Design review of the part built by this model. Coordinates are the model's own, in mm. Face numbers are marked on the shaded views. A direction names the side the tool comes from. Coordinates: 2 decimals unless noted, no trailing zeros. Loops run counter-clockwise (first coordinate to the right, second up) from the corner with the lowest first, then second, coordinate; pieces in that order, holes last. Notation, with made-up numbers: (-26.75, -22.5) -> (-9.75, -22.5) arc R31 ccw to (-9.75, 4.5) -> close; hole circle Ø2 at (35.25, 72.25). An arc over 180 degrees is marked (long way). Answer in a Markdown table with one row per item.
```python
from build123d import *

# Parameters (mm, degrees)
EXTRUDE_1_DEPTH = 20
EXTRUDE_2_DEPTH = 2.5
SKETCH_3_W      = 12
SKETCH_3_H      = 4
EXTRUDE_3_DEPTH = 10
FILLET_1_R      = 2


with BuildPart() as part:
    # 草图1 → 凸台-拉伸1 (new body)
    with BuildSketch(Plane(origin=(0, 0, 0), x_dir=(1, 0, 0), z_dir=(0, 1, 0))):
        Polygon((35, 66), (66, 35), (66, 0), (0, 0), (0, 66), align=None)
    extrude(amount=EXTRUDE_1_DEPTH)

    # 草图2 → 凸台-拉伸2 (add)
    with BuildSketch(Plane(origin=(50.5, 0, -50.5), x_dir=(-0.7071067811865475, 0, -0.7071067811865477), z_dir=(0.7071067811865477, 0, -0.7071067811865475))):
        with BuildLine():
            Line((15.5, 15), (15.5, 5))
            ThreePointArc((15.5, 5), (14.621320344, 2.878679656), (12.5, 2))
            Line((12.5, 2), (-12.5, 2))
            ThreePointArc((-12.5, 2), (-14.621320344, 2.878679656), (-15.5, 5))
            Line((-15.5, 5), (-15.5, 15))
            ThreePointArc((-15.5, 15), (-14.621320344, 17.121320344), (-12.5, 18))
            Line((-12.5, 18), (12.5, 18))
            ThreePointArc((12.5, 18), (14.621320344, 17.121320344), (15.5, 15))
        make_face()
    extrude(amount=EXTRUDE_2_DEPTH)

    # 草图3 → 凸台-拉伸3 (add)
    with BuildSketch(Plane(origin=(52.267766953, 0, -52.267766953), x_dir=(-0.7071067811865476, 0, -0.7071067811865476), z_dir=(0.7071067811865476, 0, -0.7071067811865476))):
        with Locations((0, 10)):
            Rectangle(SKETCH_3_W, SKETCH_3_H)
    extrude(amount=EXTRUDE_3_DEPTH)

    # 圆角1
    fillet_1_edges = [part.edges().sort_by_distance(p)[0] for p in [
        (66, 20, -17.5),
        (50.5, 20, -50.5),
        (17.5, 20, -66),
        (0, 20, -33),
        (17.5, 0, -66),
        (50.5, 0, -50.5),
        (66, 0, -17.5),
        (33, 0, 0),
        (0, 0, -33),
        (33, 20, 0),
        (0, 10, -66),
        (66, 10, 0),
        (0, 10, 0),
    ]]
    fillet(fillet_1_edges, radius=FILLET_1_R - 0.0001)  # a hair under: the kernel refuses the full size


solid = part.part
```
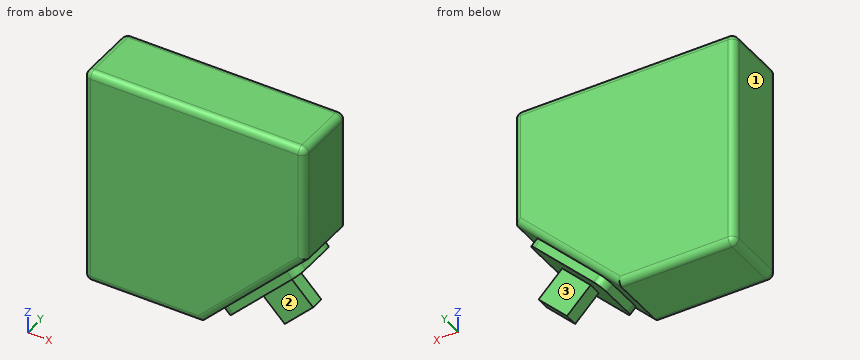
(1) Take a section at B-B on y = 13.5. Give the boundary of the cut face in (x, z), and give its area (3 significant figures).
Evaluation:
| item | result |
|---|---|
| outline | (0, -64) arc R2 ccw to (2, -66) -> (35, -66) -> (39.54, -61.46) -> (41.31, -63.23) -> (63.23, -41.31) -> (61.46, -39.54) -> (66, -35) -> (66, -2) arc R2 ccw to (64, 0) -> (2, 0) arc R2 ccw to (0, -2) -> close |
| area | 3,950 mm² |
(2) Tool access review of the marked faces 1, 2 and 3: name each direction out of +Z, -Z, +X, -X, +Y, -Y from which nothing blocks a thin tool from reaching the whole face with its end or side.
Evaluation:
| item | result |
|---|---|
| face 1 | +Z, -Z, -X, +Y, -Y |
| face 2 | -Z, +X, -Y |
| face 3 | -Z, +X, +Y |
(3) To check wall thickness, follow probe 1 along X at (y, z) = (13, -62.5); probe 2 along X at (y, z) = (1.5, -20); probe 3 along X at (y, z) = (16.5, -54). State the ranges of each line that lie inside material, in increasing order.
Evaluation:
| item | result |
|---|---|
| probe 1 | x = 0 to 38.5, 40.58 to 42.04 |
| probe 2 | x = 0.06 to 65.94 |
| probe 3 | x = 0 to 50.54 |
(4) Take a section at C-C on y = 3.25. Give the boundary of the cut face in (x, z).
Evaluation:
| item | result |
|---|---|
| outline | (0, -64) arc R2 ccw to (2, -66) -> (35, -66) -> (39.94, -61.06) -> (41.71, -62.83) -> (62.83, -41.71) -> (61.06, -39.94) -> (66, -35) -> (66, -2) arc R2 ccw to (64, 0) -> (2, 0) arc R2 ccw to (0, -2) -> close |
(5) Take a section at A-A on y = 9.5. Give the boundary of the cut face in (x, z).
Evaluation:
| item | result |
|---|---|
| outline | (0, -64) arc R2 ccw to (2, -66) -> (35, -66) -> (39.54, -61.46) -> (41.31, -63.23) -> (48.03, -56.51) -> (55.1, -63.58) -> (63.58, -55.1) -> (56.51, -48.03) -> (63.23, -41.31) -> (61.46, -39.54) -> (66, -35) -> (66, -2) arc R2 ccw to (64, 0) -> (2, 0) arc R2 ccw to (0, -2) -> close |
(6) For pin 1 (1 mm diameter, centred on x = 36, y = 14.5, fed in from -Z); pin 2 (4.5 mm diameter, centred on x = 58.5, z = -57, fed in from +Y); pin 3 (4.5 mm diameter, centred on x = 59.5, z = -59, fed in from -Y), all flat-tipped, find the tip position at first contact; note any pin that passes through.
Evaluation:
| item | result |
|---|---|
| pin 1 | stops at z = -65.5 |
| pin 2 | stops at y = 12 |
| pin 3 | stops at y = 8 |
